Source: CAD feature listing. Evaluate the final solid. Frame: model axes, mm. Face numbers are marked on the shaded views. A direction names the side the tool comes from. Coordinates: 2 decimals unless noted, no trailing zeros. Loops run counter-clockwise (first coordinate to the right, second up) from the corner with the lowest first, then second, coordinate; pieces in that order, holes last. Notation, with made-up numbers: M 76.5,-24.75 L 113.5,-24.75 A23 cw 113.5,-4.75 Z; hole C -18,21 d11. An arc over 180 degrees is marked long. One line per question, with ' | ' between items. Start each with the question number.
1. Section query D-D, the plane z = 2.3. State how many separate pieces and enclosed holes the cut face has, and give its area (3 significant figures).
2. Ray query, probe 1 along Y at (x, z) = (1.5, 2.7); probe 2 along X at (y, z) = (-21.5, 1.55); probe 3 along X at (y, z) = (24, 2.7). Return the intervals inside material, ascending.
3. Mould query, pull axis X, two halves, no side actions, for the marked faces 1, 2 and 3. Classes: pulls with the +X half, pulls with the -X half, needs draft (parallel to the pull), parting line crosses it, or undercut.
4. Section query C-C, the plane y = 26.5. Output: boundary loops of the cut face in (x, z), and give its area (3 significant figures).
5. Pin query (flat end, axial travel): P1, Ø3.5, axis at x = 14, y = 0, coming from the +Z side; P2, Ø2.5, axis at x = -2, z = 3, coming from the -Y side. Return the tip coordinate at first contact, or that it passes through.
6. Access query for the marked faces 4, 5 and 6. Directions: +Z, -Z, +X, -X, +Y, -Y. A direction counts if a zero-diameter tool reaches every point of the face in a straight line with its end or side. Return the directions, or none.
7. Section query B-B, the plane y = 10. Output: boundary loops of the cut face in (x, z), and give its area (3 significant figures).
8. Section query A-A, the plane x = -2.5. Output: boundary loops of the cut face in (y, z).
```python
from build123d import *

# Parameters (mm, degrees)
SKETCH_1_W          = 35
SKETCH_1_H          = 60
EXTRUDE_1_DEPTH     = 5
SKETCH_2_R          = 1.5
SKETCH_2_R_2        = 0.5
SKETCH_2_W          = 20
SKETCH_2_H          = 10
CUT_EXTRUDE_1_DEPTH = 36.089172119
SKETCH_3_R          = 1.5
CUT_EXTRUDE_2_DEPTH = 47.368092477
HOLE_WIZARD_M3_1_D  = 2.5
CHAMFER_1_SIZE      = 0.5


with BuildPart() as part:
    # 草图1 → 凸台-拉伸1 (new body)
    with BuildSketch(Plane.XY):
        Rectangle(SKETCH_1_W, SKETCH_1_H)
    extrude(amount=EXTRUDE_1_DEPTH)

    # 草图2 → 切除-拉伸1 (cut, through all)
    with BuildSketch(Plane.XY.offset(5)):
        with Locations((-14, 0)):
            Circle(SKETCH_2_R)
        with Locations((-14, -15)):
            Circle(SKETCH_2_R)
        with Locations(Location((14, -15, 0), (0, 0, 180))):
            Circle(SKETCH_2_R)
        with Locations(Location((14, 0, 0), (0, 0, 180))):
            Circle(SKETCH_2_R)
        with Locations((-14, -10)):
            Circle(SKETCH_2_R)
        with Locations((-13.9, -22)):
            Circle(SKETCH_2_R)
        with Locations(Location((13.9, -22, 0), (0, 0, 180))):
            Circle(SKETCH_2_R)
        with Locations(Location((14, -10, 0), (0, 0, 180))):
            Circle(SKETCH_2_R)
        with Locations(Location((-13.9, 22, 0), (0, 0, 180))):
            Circle(SKETCH_2_R)
        with Locations((13.9, 22)):
            Circle(SKETCH_2_R)
        with Locations((14, 10)):
            Circle(SKETCH_2_R)
        with Locations(Location((-14, 10, 0), (0, 0, 180))):
            Circle(SKETCH_2_R)
        with Locations((14, 15)):
            Circle(SKETCH_2_R)
        with Locations(Location((-14, 15, 0), (0, 0, 180))):
            Circle(SKETCH_2_R)
        with Locations((-5, 0)):
            Circle(SKETCH_2_R_2)
        with Locations((5, 0)):
            Circle(SKETCH_2_R_2)
        with Locations((-14, -5)):
            Circle(SKETCH_2_R)
        with Locations(Location((14, -5, 0), (0, 0, 180))):
            Circle(SKETCH_2_R)
        with Locations((14, 5)):
            Circle(SKETCH_2_R)
        with Locations(Location((-14, 5, 0), (0, 0, 180))):
            Circle(SKETCH_2_R)
        with Locations((-5, 17)):
            Circle(SKETCH_2_R_2)
        with Locations((5, 17)):
            Circle(SKETCH_2_R_2)
        with Locations(Location((5, -17, 0), (0, 0, 180))):
            Circle(SKETCH_2_R_2)
        with Locations(Location((-5, -17, 0), (0, 0, 180))):
            Circle(SKETCH_2_R_2)
        with Locations((0, 25)):
            Rectangle(SKETCH_2_W, SKETCH_2_H)
        with Locations((0, -25)):
            Rectangle(SKETCH_2_W, SKETCH_2_H)
        with BuildLine():
            Line((10, 11), (10, 6))
            ThreePointArc((10, 6), (9.121320344, 3.878679656), (7, 3))
            Line((7, 3), (-7, 3))
            ThreePointArc((-7, 3), (-9.121320344, 3.878679656), (-10, 6))
            Line((-10, 6), (-10, 11))
            ThreePointArc((-10, 11), (-9.121320344, 13.121320344), (-7, 14))
            Line((-7, 14), (7, 14))
            ThreePointArc((7, 14), (9.121320344, 13.121320344), (10, 11))
        make_face()
        with BuildLine():
            Line((-7, -14), (7, -14))
            ThreePointArc((7, -14), (9.121320344, -13.121320344), (10, -11))
            Line((10, -11), (10, -6))
            ThreePointArc((10, -6), (9.121320344, -3.878679656), (7, -3))
            Line((7, -3), (-7, -3))
            ThreePointArc((-7, -3), (-9.121320344, -3.878679656), (-10, -6))
            Line((-10, -6), (-10, -11))
            ThreePointArc((-10, -11), (-9.121320344, -13.121320344), (-7, -14))
        make_face()
    extrude(amount=-CUT_EXTRUDE_1_DEPTH, mode=Mode.SUBTRACT)

    # 草图3 → 切除-拉伸2 (cut, through all)
    with BuildSketch(Plane(origin=(17.5, 0, 0), x_dir=(0, 0, -1), z_dir=(1, 0, 0))):
        with Locations((-2.5, -26.5)):
            Circle(SKETCH_3_R)
        with Locations((-2.5, 26.5)):
            Circle(SKETCH_3_R)
    extrude(amount=-CUT_EXTRUDE_2_DEPTH, mode=Mode.SUBTRACT)

    # M3 螺纹孔1 (through all)
    with Locations(Plane.XY.offset(5)):
        with Locations((-5, 17), (5, 17), (-5, 0), (5, 0), (-5, -17), (5, -17)):
            Hole(HOLE_WIZARD_M3_1_D / 2)

    # 倒角1
    chamfer_1_edges = [part.edges().sort_by_distance(p)[0] for p in [
        (-15.5, -5, 0),
        (-15.5, -5, 5),
        (15.5, -5, 0),
        (15.5, -5, 5),
        (12.5, 5, 0),
        (12.5, 5, 5),
        (-12.5, 5, 0),
        (-12.5, 5, 5),
        (-17.5, -26.5, 4),
        (17.5, -26.5, 4),
        (-17.5, 26.5, 4),
        (17.5, 26.5, 4),
        (6.25, -17, 5),
        (6.25, -17, 0),
        (-3.75, -17, 5),
        (-3.75, -17, 0),
        (6.25, 0, 5),
        (6.25, 0, 0),
        (-3.75, 0, 5),
        (-3.75, 0, 0),
        (6.25, 17, 5),
        (6.25, 17, 0),
        (-3.75, 17, 5),
        (-3.75, 17, 0),
        (-15.5, 0, 0),
        (-15.5, 0, 5),
        (-15.5, -15, 0),
        (-15.5, -15, 5),
        (15.5, -15, 0),
        (15.5, -15, 5),
        (15.5, 0, 0),
        (15.5, 0, 5),
        (-15.5, -10, 0),
        (-15.5, -10, 5),
        (-15.4, -22, 0),
        (-15.4, -22, 5),
        (15.4, -22, 0),
        (15.4, -22, 5),
        (15.5, -10, 0),
        (15.5, -10, 5),
        (-12.4, 22, 0),
        (-12.4, 22, 5),
        (12.4, 22, 0),
        (12.4, 22, 5),
        (12.5, 10, 0),
        (12.5, 10, 5),
        (-12.5, 10, 0),
        (-12.5, 10, 5),
        (12.5, 15, 5),
        (-12.5, 15, 0),
        (-12.5, 15, 5),
    ]]
    chamfer(chamfer_1_edges, length=CHAMFER_1_SIZE)


solid = part.part
```
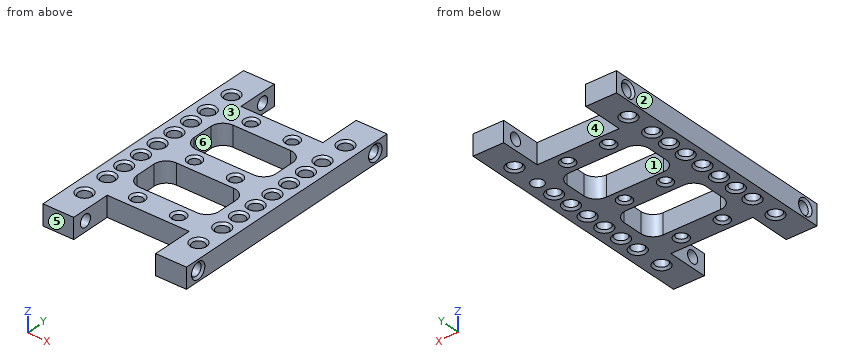
Taken from the geometry:
1) separate pieces: 5 | enclosed holes: 26 | area: 1,030 mm^2
2) probe 1: -20 to -14, -3 to 3, 14 to 20 | probe 2: -17.5 to -15.31, -12.49 to -10, 10 to 12.49, 15.31 to 17.5 | probe 3: -17.5 to -10, 10 to 17.5
3) face 1: undercut | face 2: pulls with the -X half | face 3: needs draft
4) outline: M -17.5,0 L -10,0 L -10,1 L -17,1 L -17.5,0.5 Z; M -17.5,4.5 L -17,4 L -10,4 L -10,5 L -17.5,5 Z; M 10,0 L 17.5,0 L 17.5,0.5 L 17,1 L 10,1 Z; M 10,4 L 17,4 L 17.5,4.5 L 17.5,5 L 10,5 Z | area: 29.5 mm^2
5) P1: z = 4.75 | P2: y = -20
6) face 4: +Z, -Z, +Y | face 5: +Z, -Z, +X, -X, -Y | face 6: +Z, -Z
7) outline: M -17.5,0 L -16,0 L -15.5,0.5 L -15.5,4.5 L -16,5 L -17.5,5 Z; M -12.5,0.5 L -12,0 L -10,0 L -10,5 L -12,5 L -12.5,4.5 Z; M 10,0 L 12,0 L 12.5,0.5 L 12.5,4.5 L 12,5 L 10,5 Z; M 15.5,0.5 L 16,0 L 17.5,0 L 17.5,5 L 16,5 L 15.5,4.5 Z | area: 44.0 mm^2
8) outline: M -20,0 L -14,0 L -14,5 L -20,5 Z; M -3,0 L 3,0 L 3,5 L -3,5 Z; M 14,0 L 20,0 L 20,5 L 14,5 Z
